For this review, take the finished solid that the model builds, in its own axes (mm). A direction names the side the tool comes from. Round coordinates to 2 decimals unless told otherwise and drop trailing zeros. Write each loop counter-clockwise with the first axis right and the second up, starting at its lowest first coordinate (ties: lowest second). Pieces come first, ordered by that corner, then holes. Notation, with made-up numbers: M 79,34 L 89,34 A18 cw 89,44 Z; hole C 7,35 d8. An arc over 180 degrees is marked long. One line per question, with ' | ' between items.
```python
from build123d import *

# Parameters (mm, degrees)
SKETCH2_W               = 279.4
SKETCH2_H               = 127
BOSS_EXTRUDE1_DEPTH     = 9.525
SKETCH3_W               = 25.4
SKETCH3_H               = 9.525
BOSS_EXTRUDE2_DEPTH     = 9.525
LPATTERN1_COUNT         = 6
LPATTERN1_PITCH         = 50.8
MIRROR1_COPY_1_SKETCH_W = 25.4
MIRROR1_COPY_1_SKETCH_H = 9.525
MIRROR1_COPY_1_DEPTH    = 9.525
MIRROR1_COPY_2_SKETCH_W = 25.4
MIRROR1_COPY_2_SKETCH_H = 9.525
MIRROR1_COPY_2_DEPTH    = 9.525
MIRROR1_COPY_3_SKETCH_W = 25.4
MIRROR1_COPY_3_SKETCH_H = 9.525
MIRROR1_COPY_3_DEPTH    = 9.525
MIRROR1_COPY_4_SKETCH_W = 25.4
MIRROR1_COPY_4_SKETCH_H = 9.525
MIRROR1_COPY_4_DEPTH    = 9.525
MIRROR1_COPY_5_SKETCH_W = 25.4
MIRROR1_COPY_5_SKETCH_H = 9.525
MIRROR1_COPY_5_DEPTH    = 9.525
SKETCH4_W               = 25.4
SKETCH4_H               = 9.525
BOSS_EXTRUDE3_DEPTH     = 9.525
LPATTERN2_COUNT         = 3
LPATTERN2_PITCH         = 50.8
MIRROR2_COPY_1_SKETCH_W = 25.4
MIRROR2_COPY_1_SKETCH_H = 9.525
MIRROR2_COPY_1_DEPTH    = 9.525
MIRROR2_COPY_2_SKETCH_W = 25.4
MIRROR2_COPY_2_SKETCH_H = 9.525
MIRROR2_COPY_2_DEPTH    = 9.525
SKETCH6_W               = 9.525
SKETCH6_H               = 9.525
BOSS_EXTRUDE4_DEPTH     = 9.525
MIRROR4_COPY_1_SKETCH_W = 9.525
MIRROR4_COPY_1_SKETCH_H = 9.525
MIRROR4_COPY_1_DEPTH    = 9.525
MIRROR4_COPY_2_SKETCH_W = 9.525
MIRROR4_COPY_2_SKETCH_H = 9.525
MIRROR4_COPY_2_DEPTH    = 9.525


with BuildPart() as part:
    # Sketch2 → Boss-Extrude1 (new body)
    with BuildSketch(Plane(origin=(0, 0, 0), x_dir=(1, 0, 0), z_dir=(0, 1, 0))):
        Rectangle(SKETCH2_W, SKETCH2_H)
    extrude(amount=BOSS_EXTRUDE1_DEPTH)

    # Sketch3 → Boss-Extrude2 (add)
    with BuildSketch(Plane.XY.offset(63.5)):
        with Locations((-127, 4.7625)):
            Rectangle(SKETCH3_W, SKETCH3_H)
    boss_extrude2 = extrude(amount=BOSS_EXTRUDE2_DEPTH)

    # LPattern1: Boss-Extrude2 ×6
    with Locations(*[(i * LPATTERN1_PITCH, 0, 0) for i in range(1, LPATTERN1_COUNT)]):
        add(boss_extrude2)

    # Mirror1: Boss-Extrude2 across plane
    add(boss_extrude2.mirror(Plane.XY))

    # Mirror1 copy 1 sketch → Mirror1 copy 1 (add)
    with BuildSketch(Plane(origin=(50.8, 0, -63.5), x_dir=(1, 0, 0), z_dir=(0, 0, -1))):
        with Locations((-127, -4.7625)):
            Rectangle(MIRROR1_COPY_1_SKETCH_W, MIRROR1_COPY_1_SKETCH_H)
    extrude(amount=MIRROR1_COPY_1_DEPTH)

    # Mirror1 copy 2 sketch → Mirror1 copy 2 (add)
    with BuildSketch(Plane(origin=(101.6, 0, -63.5), x_dir=(1, 0, 0), z_dir=(0, 0, -1))):
        with Locations((-127, -4.7625)):
            Rectangle(MIRROR1_COPY_2_SKETCH_W, MIRROR1_COPY_2_SKETCH_H)
    extrude(amount=MIRROR1_COPY_2_DEPTH)

    # Mirror1 copy 3 sketch → Mirror1 copy 3 (add)
    with BuildSketch(Plane(origin=(152.4, 0, -63.5), x_dir=(1, 0, 0), z_dir=(0, 0, -1))):
        with Locations((-127, -4.7625)):
            Rectangle(MIRROR1_COPY_3_SKETCH_W, MIRROR1_COPY_3_SKETCH_H)
    extrude(amount=MIRROR1_COPY_3_DEPTH)

    # Mirror1 copy 4 sketch → Mirror1 copy 4 (add)
    with BuildSketch(Plane(origin=(203.2, 0, -63.5), x_dir=(1, 0, 0), z_dir=(0, 0, -1))):
        with Locations((-127, -4.7625)):
            Rectangle(MIRROR1_COPY_4_SKETCH_W, MIRROR1_COPY_4_SKETCH_H)
    extrude(amount=MIRROR1_COPY_4_DEPTH)

    # Mirror1 copy 5 sketch → Mirror1 copy 5 (add)
    with BuildSketch(Plane(origin=(254, 0, -63.5), x_dir=(1, 0, 0), z_dir=(0, 0, -1))):
        with Locations((-127, -4.7625)):
            Rectangle(MIRROR1_COPY_5_SKETCH_W, MIRROR1_COPY_5_SKETCH_H)
    extrude(amount=MIRROR1_COPY_5_DEPTH)

    # Sketch4 → Boss-Extrude3 (add)
    with BuildSketch(Plane(origin=(139.7, 0, 0), x_dir=(0, 0, -1), z_dir=(1, 0, 0))):
        with Locations((-50.8, 4.7625)):
            Rectangle(SKETCH4_W, SKETCH4_H)
    boss_extrude3 = extrude(amount=BOSS_EXTRUDE3_DEPTH)

    # LPattern2: Boss-Extrude3 ×3
    with Locations(*[(0, 0, -i * LPATTERN2_PITCH) for i in range(1, LPATTERN2_COUNT)]):
        add(boss_extrude3)

    # Mirror2: Boss-Extrude3 across plane
    add(boss_extrude3.mirror(Plane(origin=(0, 0, 0), x_dir=(0, 0, 1), z_dir=(1, 0, 0))))

    # Mirror2 copy 1 sketch → Mirror2 copy 1 (add)
    with BuildSketch(Plane(origin=(-139.7, 0, -50.8), x_dir=(0, 0, -1), z_dir=(-1, 0, 0))):
        with Locations((-50.8, -4.7625)):
            Rectangle(MIRROR2_COPY_1_SKETCH_W, MIRROR2_COPY_1_SKETCH_H)
    extrude(amount=MIRROR2_COPY_1_DEPTH)

    # Mirror2 copy 2 sketch → Mirror2 copy 2 (add)
    with BuildSketch(Plane(origin=(-139.7, 0, -101.6), x_dir=(0, 0, -1), z_dir=(-1, 0, 0))):
        with Locations((-50.8, -4.7625)):
            Rectangle(MIRROR2_COPY_2_SKETCH_W, MIRROR2_COPY_2_SKETCH_H)
    extrude(amount=MIRROR2_COPY_2_DEPTH)

    # Sketch6 → Boss-Extrude4 (add)
    with BuildSketch(Plane.XY.offset(63.5)):
        with Locations((144.4625, 4.7625)):
            Rectangle(SKETCH6_W, SKETCH6_H)
    boss_extrude4 = extrude(amount=BOSS_EXTRUDE4_DEPTH)

    # Mirror3: Boss-Extrude4 across plane
    add(boss_extrude4.mirror(Plane(origin=(0, 0, 0), x_dir=(0, 0, 1), z_dir=(1, 0, 0))))

    # Mirror4 copy 1 sketch → Mirror4 copy 1 (add)
    with BuildSketch(Plane(origin=(0, 0, -63.5), x_dir=(-1, 0, 0), z_dir=(0, 0, -1))):
        with Locations((144.4625, 4.7625)):
            Rectangle(MIRROR4_COPY_1_SKETCH_W, MIRROR4_COPY_1_SKETCH_H)
    extrude(amount=MIRROR4_COPY_1_DEPTH)

    # Mirror4 copy 2 sketch → Mirror4 copy 2 (add)
    with BuildSketch(Plane(origin=(0, 0, -63.5), x_dir=(1, 0, 0), z_dir=(0, 0, -1))):
        with Locations((144.4625, -4.7625)):
            Rectangle(MIRROR4_COPY_2_SKETCH_W, MIRROR4_COPY_2_SKETCH_H)
    extrude(amount=MIRROR4_COPY_2_DEPTH)


solid = part.part
```
Item 1: Take a section at A-A (z = 29). Write out the cut boundary in (x, y) (3 decimals), then the cut area to 3 significant figures.
Results:
outline: M -139.7,0 L 139.7,0 L 139.7,9.525 L -139.7,9.525 Z | area: 2,660 mm2
Item 2: Mouldability with a two-part tool opening along X and no side actions: class faces 1 (the face through (63.5, 5, -68)), 2 (the face through (149.225, 5, 0)), 3 (the face through (-144, 5, -12.7)) as +X half, -X half, draft (parallel to the pull), parting line (faces both ways), or undercut.
Results:
face 1: undercut | face 2: +X half | face 3: draft
Item 3: Machinability: for faces 4 (the face through (101, 5, 63.5)), 5 (the face through (0, 5, -63.5)), 6 (the face through (144, 5, 12.7)), 7 (the face through (-144, 5, 38.1)), which of the approach directions +Z, -Z, +X, -X, +Y, -Y give a long, thin tool a straight path to every point of the face, cutting with its end or side? Answer none if there is none.
Results:
face 4: +Z, +Y, -Y | face 5: -Z, +Y, -Y | face 6: +X, +Y, -Y | face 7: -X, +Y, -Y
Item 4: Insertion check: pin 1 Ø3 at (y, z) = (6, 23.5) entering from -X; pin 2 Ø1 at (x, y) = (-2, 6) entering from -Z; pin 3 Ø5 at (x, y) = (103.5, 4.5) entering from +Z. Each pin has a flat end and moves straight along its axis. Give the tip position at first contact, or say it passes through.
Results:
pin 1: x = -139.7 | pin 2: z = -63.5 | pin 3: z = 63.5
Item 5: Take a section at B-B (x = -107.5). Write out the cut boundary in (y, z) (3 decimals), then the cut area to 3 significant figures.
Results:
outline: M 0,-63.5 L 9.525,-63.5 L 9.525,63.5 L 0,63.5 Z | area: 1,210 mm2
Item 6: To check wall thickness, follow line 1 along Z through (x, y) = (-5, 4); line 2 along X through (y, z) = (4, 35). State the ranges of each line that lie inside material, in increasing order. Write a range as from..to.
Results:
line 1: -63.5..63.5 | line 2: -139.7..139.7
